from build123d import *

# Parameters (mm, degrees)
SKETCH1_R           = 28.1
BOSS_EXTRUDE2_DEPTH = 61.3
SKETCH3_R           = 18.6
CUT_EXTRUDE2_DEPTH  = 58.8
SKETCH4_W           = 56.2
SKETCH4_H           = 56.2
BOSS_EXTRUDE3_DEPTH = 56.2
SKETCH5_R           = 16.1
CUT_EXTRUDE4_DEPTH  = 5
SKETCH6_W           = 49.797391422
SKETCH6_H           = 49.779255452
CUT_EXTRUDE5_DEPTH  = 53.7
SKETCH7_R           = 28.1
BOSS_EXTRUDE4_DEPTH = 321.5
CUT_EXTRUDE6_DEPTH  = 10
SKETCH9_R           = 3
CUT_EXTRUDE7_DEPTH  = 1
SKETCH10_R          = 6.025
CUT_EXTRUDE8_DEPTH  = 0.1
SKETCH18_R          = 3.75
CUT_EXTRUDE9_DEPTH  = 100
SKETCH19_R          = 3.75
CUT_EXTRUDE11_DEPTH = 325
SKETCH20_W          = 56.2
SKETCH20_H          = 56.2
CUT_EXTRUDE13_DEPTH = 200
SKETCH22_R          = 28.332078896
CUT_EXTRUDE15_DEPTH = 171.5


with BuildPart() as part:
    # Sketch1 → Boss-Extrude2 (new body)
    with BuildSketch(Plane.XY):
        Circle(SKETCH1_R)
    extrude(amount=BOSS_EXTRUDE2_DEPTH)

    # Sketch3 → Cut-Extrude2 (cut)
    with BuildSketch(Plane.XY.offset(61.3)):
        with Locations((0, -7)):
            Circle(SKETCH3_R)
    extrude(amount=-CUT_EXTRUDE2_DEPTH, mode=Mode.SUBTRACT)

    # Sketch4 → Boss-Extrude3 (add)
    with BuildSketch(Plane(origin=(0, 0, 0), x_dir=(-1, 0, 0), z_dir=(0, 0, -1))):
        Rectangle(SKETCH4_W, SKETCH4_H)
    extrude(amount=BOSS_EXTRUDE3_DEPTH)

    # Sketch5 → Cut-Extrude4 (cut)
    with BuildSketch(Plane.XY.offset(2.5)):
        with Locations((0, -7)):
            Circle(SKETCH5_R)
    extrude(amount=-CUT_EXTRUDE4_DEPTH, mode=Mode.SUBTRACT)

    # Sketch6 → Cut-Extrude5 (cut)
    with BuildSketch(Plane(origin=(0, 0, -56.2), x_dir=(-1, 0, 0), z_dir=(0, 0, -1))):
        Rectangle(SKETCH6_W, SKETCH6_H)
    extrude(amount=-CUT_EXTRUDE5_DEPTH, mode=Mode.SUBTRACT)

    # Sketch7 → Boss-Extrude4 (add)
    with BuildSketch(Plane(origin=(0, -28.1, 0), x_dir=(-1, 0, 0), z_dir=(0, -1, 0))):
        with Locations(Location((0, 28.1, 0), (0, 0, 90))):
            Circle(SKETCH7_R)
    extrude(amount=BOSS_EXTRUDE4_DEPTH)

    # Sketch8 → Cut-Extrude6 (cut)
    with BuildSketch(Plane(origin=(0, -349.6, 0), x_dir=(-1, 0, 0), z_dir=(0, -1, 0))):
        with BuildLine():
            Line((-1.658312395, 25.832078896), (1.658312395, 25.832078896))
            ThreePointArc((1.658312395, 25.832078896), (3, 28.332078896), (1.658312395, 30.832078896))
            Line((1.658312395, 30.832078896), (-1.658312395, 30.832078896))
            ThreePointArc((-1.658312395, 30.832078896), (-3, 28.332078896), (-1.658312395, 25.832078896))
        make_face()
    extrude(amount=-CUT_EXTRUDE6_DEPTH, mode=Mode.SUBTRACT)

    # Sketch9 → Cut-Extrude7 (cut)
    with BuildSketch(Plane(origin=(0, -349.6, 0), x_dir=(-1, 0, 0), z_dir=(0, -1, 0))):
        with Locations(Location((0, 28.332078896, 0), (0, 0, 90))):
            Circle(SKETCH9_R)
    extrude(amount=-CUT_EXTRUDE7_DEPTH, mode=Mode.SUBTRACT)

    # Sketch10 → Cut-Extrude8 (cut)
    with BuildSketch(Plane(origin=(0, -349.6, 0), x_dir=(-1, 0, 0), z_dir=(0, -1, 0))):
        with Locations(Location((0, 28.332078896, 0), (0, 0, 90))):
            Circle(SKETCH10_R)
    extrude(amount=-CUT_EXTRUDE8_DEPTH, mode=Mode.SUBTRACT)

    # Cut-Sweep4: sweep along a path in Sketch15
    with BuildLine(Plane(origin=(0, -349.6, 0), x_dir=(-1, 0, 0), z_dir=(0, -1, 0))) as cut_sweep4_path:
        ThreePointArc((15, 28.332078896), (0, 43.332078896), (-15, 28.332078896))
    # 3DSketch2 → Cut-Sweep4 (sweep, cut)
    with BuildSketch(Plane(origin=(-15, -349.6, -28.332078896), x_dir=(-0.022748965612757834, 0.999741208795331, 0), z_dir=(0, 0, 1))):
        Polygon((0, 0), (0.170617242, 7.498059066), (329.685319661, 0), (329.514702419, -7.498059066), align=None)
    sweep(path=cut_sweep4_path.line, mode=Mode.SUBTRACT)

    # Sketch18 → Cut-Extrude9 (cut)
    with BuildSketch(Plane.XY.offset(61.3)):
        with Locations((0, 18.75)):
            Circle(SKETCH18_R)
    extrude(amount=-CUT_EXTRUDE9_DEPTH, mode=Mode.SUBTRACT)

    # Sketch19 → Cut-Extrude11 (cut)
    with BuildSketch(Plane(origin=(0, -349.6, 0), x_dir=(-1, 0, 0), z_dir=(0, -1, 0))):
        with Locations((-18.75, 28.332078896)):
            Circle(SKETCH19_R)
        with Locations((18.75, 28.332078896)):
            Circle(SKETCH19_R)
    extrude(amount=-CUT_EXTRUDE11_DEPTH, mode=Mode.SUBTRACT)

    # Sketch20 → Cut-Extrude13 (cut)
    with BuildSketch(Plane(origin=(0, 0, -56.2), x_dir=(-1, 0, 0), z_dir=(0, 0, -1))):
        Rectangle(SKETCH20_W, SKETCH20_H)
    extrude(amount=-CUT_EXTRUDE13_DEPTH, mode=Mode.SUBTRACT)

    # Sketch22 → Cut-Extrude15 (cut)
    with BuildSketch(Plane(origin=(0, -349.6, 0), x_dir=(-1, 0, 0), z_dir=(0, -1, 0))):
        with Locations((0, 28.332078896)):
            Circle(SKETCH22_R)
    extrude(amount=-CUT_EXTRUDE15_DEPTH, mode=Mode.SUBTRACT)


solid = part.part
Here's how the part is built. I have some questions about the finished solid (model axes, mm). A direction names the side the tool comes from. Round coordinates to 2 decimals unless told otherwise and drop trailing zeros. Order: outer loops, then holes, each group sorted by start corner. A loop starts at its lowest first (then second) coordinate and runs counter-clockwise, first axis right, second up. Notation, with made-up numbers: (14, -13.5) -> (64, -13.5) arc R15 cw to (64, 15.5) -> close; hole circle Ø8 at (31, 60.5). An arc over 180 degrees is marked (long way). Use CSV: the item, a comma, the result in double quotes.
1. I want a section at B-B on z = -34.5. List the corners of the cut face in (x, y) for me.
Recorded:
outline,"(-27.36, -178.1) -> (-21.64, -178.1) -> (-21.64, -28.1) -> (-27.36, -28.1) -> close; (-13.67, -178.1) -> (13.67, -178.1) -> (13.67, -28.1) -> (-13.67, -28.1) -> close; (21.64, -178.1) -> (27.36, -178.1) -> (27.36, -28.1) -> (21.64, -28.1) -> close"
2. I need wall thicknesses on line 1 along X through (y, z) = (-47, -35); line 2 along X through (y, z) = (-146, -38); line 3 along Z through (x, y) = (0.5, -71). Which ranges of each line are inside material? Lowest first, please.
Recorded:
line 1,"x = -27.24 to -21.49, -13.44 to 13.44, 21.49 to 27.24"
line 2,"x = -26.3 to -20.32, -11.47 to 11.47, 20.32 to 26.3"
line 3,"z = -56.2 to -50.83, -43.32 to 0"
3. Which directions (+Z, -Z, +X, -X, +Y, -Y) give clear straight access to the entire face, cutting with the end or side of a thin tool? Please do faces 1 (the face through (0, -178.1, -22)), 2 (the face through (-0.33, -102.05, -43.33)).
Recorded:
face 1,"+Z, -Z, +X, -X, -Y"
face 2,"+Y, -Y"
4. Thinking about a two-plate mould opening in Z: for faces 3 (the face through (-10.76, -102.05, -54.06)), 4 (the face through (18.832, -104.15, -24.583)), 5 (the face through (0, -28.1, -22)), which applies, pulls with the +Z half, pulls with the -Z half, needs draft (parallel to the pull), parting line crosses it, or undercut?
Recorded:
face 3,"parting line crosses it"
face 4,"undercut"
face 5,"needs draft"
5. I'm going to push flat-ended pins straight in: P1, Ø8, axis at y = -141.5, z = -48.5, coming from the +X side; P2, Ø5, axis at y = -90, z = -50.5, coming from the +X side; P3, Ø10, axis at y = -77, z = -47, coming from the +X side. Where does each tip first touch, or does it pass through?
Recorded:
P1,"stops at x = 22.82"
P2,"stops at x = 19.84"
P3,"stops at x = 24.42"
6. I want a section at C-C on z = -48.5. List the corners of the cut face in (x, y) for me.
Recorded:
outline,"(-19.32, -178.1) -> (-9.98, -178.1) -> (-9.98, -28.1) -> (-19.32, -28.1) -> close; (9.98, -178.1) -> (19.32, -178.1) -> (19.32, -28.1) -> (9.98, -28.1) -> close"
7. I want a section at D-D on y = -107. List the corners of the cut face in (x, z) for me, and give its area (3 significant figures).
Recorded:
outline,"circle Ø56.2 at (0, -28.1); hole (-22.5, -28.33) arc R22.5 ccw to (22.5, -28.33) arc R3.75 ccw to (15, -28.33) arc R15 cw to (-15, -28.33) arc R3.75 ccw to start"
area,"1,990 mm2"
8. I want a section at A-A on x = 0. List the corners of the cut face in (y, z) for me.
Recorded:
outline,"(-178.1, -56.2) -> (-28.1, -56.2) -> (-28.1, -50.83) -> (-178.1, -50.83) -> close; (-178.1, -43.33) -> (-28.1, -43.33) -> (-28.1, 0) -> (-178.1, 0) -> close"
